from build123d import *
from build123d import SkipClean  # not in build123d's __all__

# Parameters (mm, degrees)
F0_R     = 4
F1_DEPTH = 2.54


with BuildPart() as f1:
    # F0 (on Top) → F1 (new body, symmetric)
    with BuildSketch(Plane.XY):
        with BuildLine():
            Line((12.7523779158, 9.5117846914), (-2.9762470444, 32.0985170452))
            ThreePointArc((-2.9762470444, 32.0985170452), (-14.6529201579, 43.7315272534), (-18.9402122051, 27.8164165593))
            Line((-18.9402122051, 27.8164165593), (-18.9402122051, 0))
            Line((-18.9402122051, 0), (-11.187657958, 0))
            Line((-11.187657958, 0), (-11.187657958, 18.4020288289))
            ThreePointArc((-11.187657958, 18.4020288289), (-9.1615879854, 21.1358961189), (-5.9564906022, 19.9929435136))
            Line((-5.9564906022, 19.9929435136), (4.1191245614, 4.9599822668))
            ThreePointArc((4.1191245614, 4.9599822668), (3.0807470851, 2.5759836915), (2.725803411, 0))
            Line((2.725803411, 0), (8.250803411, 0))
            ThreePointArc((8.250803411, 0), (12.250803411, 4), (16.250803411, 0))
            Line((16.250803411, 0), (21.775803411, 0))
            ThreePointArc((21.775803411, 0), (19.1610538463, 6.5554606185), (12.7523779158, 9.5117846914))
        make_face()
        with Locations((-12.1852122247, 34.5317423344)):
            Circle(F0_R, mode=Mode.SUBTRACT)
    extrude(amount=F1_DEPTH, both=True)

    # F2: F1 across plane


with BuildPart() as f1_1:
    add(f1.part, clean=False)
    with SkipClean():  # cleaning this boolean's faces spoils the solid; the shape is the same uncleaned
        add(f1.part.mirror(Plane.XZ), clean=False)


solid = f1_1.part
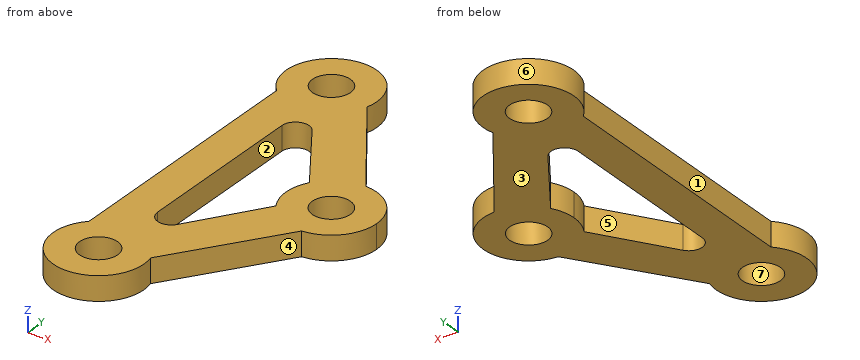
Here's how the part is built. I have some questions about the finished solid (model axes, mm). Face numbers are marked on the shaded views. A direction names the side the tool comes from. Coordinates: 2 decimals unless noted, no trailing zeros. Write each loop counter-clockwise with the first axis right and the second up, starting at its lowest first coordinate (ties: lowest second). Pieces come first, ordered by that corner, then holes.
Item 1: Will these pins go through, and if not, where does the flat tip stop? pin 1 (7 mm diameter, centred on x = 12.25, y = 0, fed in from -Z); pin 2 (1.5 mm diameter, centred on x = -1, z = 1, fed in from +Y); pin 3 (3 mm diameter, centred on x = 15.5, z = 1, fed in from -Y); pin 4 (1.5 mm diameter, centred on y = 5.5, z = 1, fed in from -X).
Item 2: If we mould it in two halves opening along X, with no side actions, what happens to the marked faces 4, 5, 6 and 7? For each: +X half, -X half, draft (parallel to the pull), parting line (faces both ways), or undercut.
Item 3: I want a section at A-A on x = 14. Write out the boundary of the cut face in (y, z).
Item 4: On a 3-axis mill with a long thin cutter (end or side, diameter ignored), from which of +Z, -Z, +X, -X, +Y, -Y can I reach the whole of each face in a straight line? I mean the marked faces 1, 2 and 3. Say none if no direction works.
Item 5: I want a section at B-B on z = 0.9. Count the separate pieces of the cut face and the enclosed holes in it, and give its area (3 significant figures).
Item 6: I want a section at C-C on y = 24. Write out the boundary of the cut face in (x, z).
Item 7: I want a section at D-D on x = 6.5. Write out the boundary of the cut face in (y, z).
Item 8: If I drill on line 1 (X direction, y = 0, z = -0.55); line 2 (Y direction, x = -10, z = -0.75); line 3 (Y direction, x = -13, z = 1.8), over which ranges is the centre line in solid material (lowest first)?
Findings below:
1. pin 1: passes through
1. pin 2: stops at y = 30.34
1. pin 3: stops at y = -9.36
1. pin 4: stops at x = -18.94
2. face 4: +X half
2. face 5: undercut
2. face 6: parting line
2. face 7: undercut
3. outline: (-9.36, -2.54) - (-3.6, -2.54) - (-3.6, 2.54) - (-9.36, 2.54) - close; (3.6, -2.54) - (9.36, -2.54) - (9.36, 2.54) - (3.6, 2.54) - close
4. face 1: +Z, -Z, -X
4. face 2: +Z, -Z
4. face 3: -Z, +X, -X, +Y, -Y
5. separate pieces: 1
5. enclosed holes: 4
5. area: 1,590 mm2
6. outline: (-18.94, -2.54) - (2.66, -2.54) - (2.66, 2.54) - (-18.94, 2.54) - close
7. outline: (-18.49, -2.54) - (18.49, -2.54) - (18.49, 2.54) - (-18.49, 2.54) - close
8. line 1: x = -18.94 to -11.19, 2.73 to 8.25, 16.25 to 21.78
8. line 2: y = -43.8 to -37.88, -31.18 to -20.72, 20.72 to 31.18, 37.88 to 43.8
8. line 3: y = -44.02 to -38.45, -30.62 to 30.62, 38.45 to 44.02
